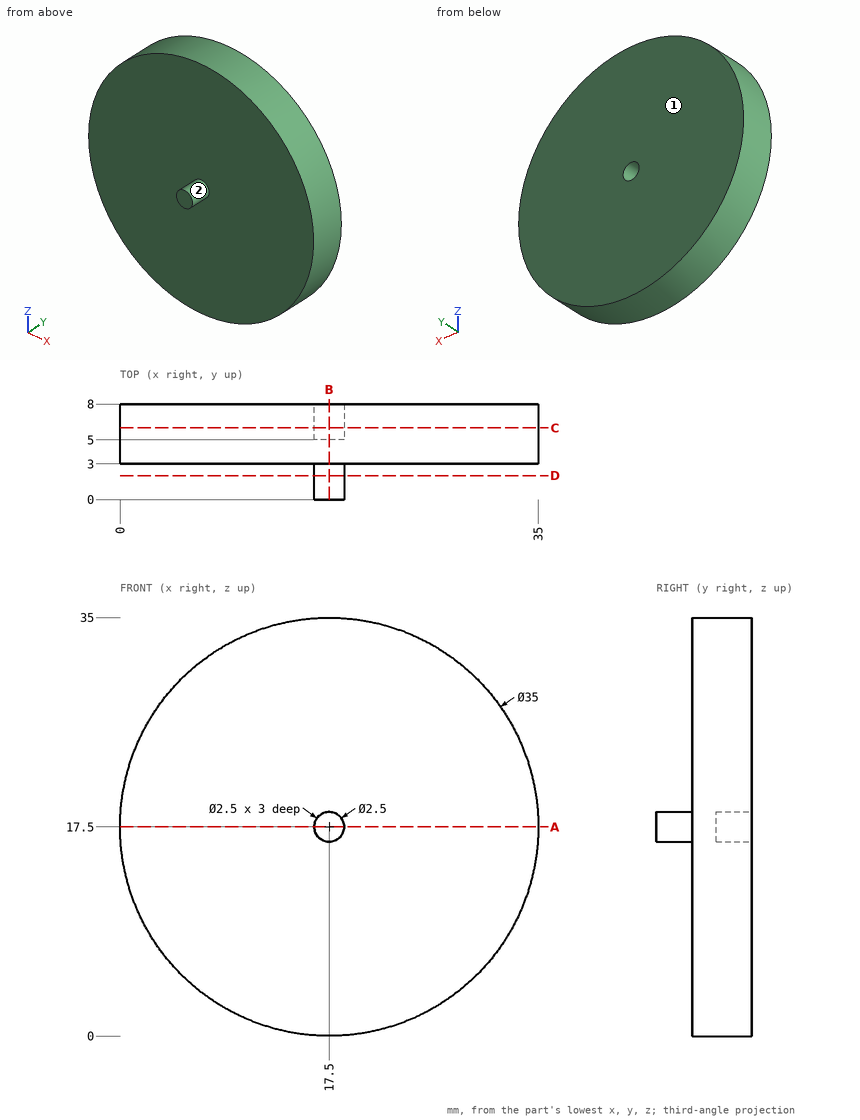
For this review, use the dimensioned drawing (mm, ordinates from the lowest corner) and the shaded views. A direction names the side the tool comes from. Coordinates: 2 decimals unless noted, no trailing zeros. Loops run counter-clockwise (first coordinate to the right, second up) from the corner with the lowest first, then second, coordinate; pieces in that order, holes last. Notation, with made-up numbers: (47.25, 30.25) -> (59.25, 30.25) arc R8 cw to (59.25, 45.25) -> close; hole circle Ø7 at (45, -2). An arc over 180 degrees is marked (long way). Use a Markdown table: item, result. Add a question column.
1. To check wall thickness, follow line 1 (X direction, y = 5.8, z = 17.5); line 2 (Y direction, x = 26, z = 18.5). State the ranges of each line that lie inside material, in increasing order.
2. Clearance check with flat-ended pins moving along their axes: pin 1 Ø4 at (x, z) = (30, 16) entering from -Y; pin 2 Ø2 at (x, y) = (13, 6.5) entering from +Z. State where each tip first meets the part, or that it passes through.
3. Add section C-C on y = 6. Write out the cut boundary in (x, z), plus the area to 3 significant figures.
4. Add section D-D on y = 2. Write out the cut boundary in (x, z), plus the area to 3 significant figures.
5. Add section B-B on x = 17.5. Write out the cut boundary in (y, z).
6. Machinability: for the marked faces 1 and 2, which of the approach directions +Z, -Z, +X, -X, +Y, -Y give a long, thin tool a straight path to every point of the face, cutting with its end or side? Answer none if there is none.
7. Add section A-A on z = 17.5. Write out the cut boundary in (x, y).
Returned:
| question | item | result |
|---|---|---|
| 1 | line 1 | x = 0 to 16.25, 18.75 to 35 |
| 1 | line 2 | y = 3 to 8 |
| 2 | pin 1 | stops at y = 3 |
| 2 | pin 2 | stops at z = 34.65 |
| 3 | outline | circle Ø35 at (17.5, 17.5); hole circle Ø2.5 at (17.5, 17.5) |
| 3 | area | 957 mm² |
| 4 | outline | circle Ø2.5 at (17.5, 17.5) |
| 4 | area | 4.91 mm² |
| 5 | outline | (0, 16.25) -> (3, 16.25) -> (3, 0) -> (8, 0) -> (8, 16.25) -> (5, 16.25) -> (5, 18.75) -> (8, 18.75) -> (8, 35) -> (3, 35) -> (3, 18.75) -> (0, 18.75) -> close |
| 6 | face 1 | +Z, -Z, +X, -X, +Y |
| 6 | face 2 | -Y |
| 7 | outline | (0, 3) -> (16.25, 3) -> (16.25, 0) -> (18.75, 0) -> (18.75, 3) -> (35, 3) -> (35, 8) -> (18.75, 8) -> (18.75, 5) -> (16.25, 5) -> (16.25, 8) -> (0, 8) -> close |
